Could you check a few things on this model? Use its own coordinates, in mm. A direction names the side the tool comes from. Coordinates: 2 decimals unless noted, no trailing zeros. Order: outer loops, then holes, each group sorted by start corner. A loop starts at its lowest first (then second) coordinate and runs counter-clockwise, first axis right, second up. Notation, with made-up numbers: (49.25, 34.25) -> (57.25, 34.25) arc R26 cw to (57.25, 57.25) -> close; hole circle Ø11 at (60, 55.5). An arc over 180 degrees is marked (long way). Put each result on its own line as item: value. Start each with the question number.
Q1. Please list where these lines run through material, in increasing order: line 1 along X through (y, z) = (31, -1.9); line 2 along X through (y, z) = (29, -0.2); line 3 along Y through (x, z) = (-52, -2.9).
Q2. We'd pull the mould along X, two halves only. Please class faces 1 (the face through (0, 15, -2)), 2 (the face through (-21.74, 14.93, -1.61)), 3 (the face through (-80, 33, 0)): +X half, -X half, draft (parallel to the pull), parting line (faces both ways), or undercut.
Q3. If we section it at C-C (z = -0.9): Count the separate pieces of the cut face and the enclosed holes in it, and give its area (3 significant figures).
Q4. For faces 4 (the face through (-26.988, 42, -2)), 5 (the face through (-58.444, 35.435, -1.61)), which set-ups out of +Z, -Z, +X, -X, +Y, -Y let a thin tool reach every point of the face, with its end or its side?
Q5. If we section it at A-A (x = -35.56): Please give me the cut outline in (y, z) (3 decimals), and give its area (3 significant figures).
Q6. Will these pins go through, and if not, where does the flat tip stop? pin 1 (1.5 mm diameter, centred on y = 23.5, z = -2.5, fed in from -X); pin 2 (1.6 mm diameter, centred on x = -9.5, z = -1.5, fed in from +Y).
Q7. If we section it at B-B (y = 50.8): Please give me the cut outline in (x, z) (3 decimals).
Q8. If we section it at D-D (x = -125.5): Please give me the cut outline in (y, z) (3 decimals).
from build123d import *

# Parameters (mm, degrees)
BOSS_EXTRUDE1_DEPTH             = 3.175
F_1_2_0_5_DIAMETER_HOLE1_D      = 12.7
F_9_64_0_14063_DIAMETER_HOLE1_D = 3.572002
F_6_CLEARANCE_HOLE1_D           = 4.3053
F_6_CLEARANCE_HOLE2_D           = 4.3053


with BuildPart() as part:
    # Sketch1 → Boss-Extrude1 (new body)
    with BuildSketch(Plane.XY):
        with BuildLine():
            Line((-26.9875, 34.925), (-26.9875, 48.5775))
            Line((-26.9875, 48.5775), (-38.29743402, 59.88743402))
            Line((-38.29743402, 59.88743402), (-157.398586801, 65.087510963))
            Line((-157.398586801, 65.087510963), (-153.9875, 1.0725e-05))
            Line((-153.9875, 1.0725e-05), (0, 0))
            Line((0, 0), (0, 30.1625))
            Line((0, 30.1625), (-22.225, 30.1625))
            ThreePointArc((-22.225, 30.1625), (-25.592596045, 31.557403955), (-26.9875, 34.925))
        make_face()
    extrude(amount=-BOSS_EXTRUDE1_DEPTH)

    # 1/2 (0.5) Diameter Hole1 (through all)
    with Locations(Plane.XY):
        with Locations((-112.7125, 33.528), (-52.3875, 33.528)):
            Hole(F_1_2_0_5_DIAMETER_HOLE1_D / 2)

    # 9/64 (0.14063) Diameter Hole1 (through all)
    with Locations(Plane.XY):
        with Locations((-112.7125, 43.053), (-52.3875, 43.053)):
            Hole(F_9_64_0_14063_DIAMETER_HOLE1_D / 2)

    # #6 Clearance Hole1 (through all)
    with Locations(Plane.XY):
        with Locations((-133.35, 30.1625), (-35.56, 43.688)):
            Hole(F_6_CLEARANCE_HOLE1_D / 2)

    # #6 Clearance Hole2 (through all)
    with Locations(Plane.XY):
        with Locations((-138.1125, 50.8), (-19.685, 14.2875)):
            Hole(F_6_CLEARANCE_HOLE2_D / 2)


solid = part.part
The answers:
1. line 1: -155.61 to -135.33, -131.37 to -118.54, -106.89 to -58.21, -46.56 to -24.92
1. line 2: -155.51 to -135.16, -131.54 to -117.16, -108.26 to -56.84, -47.94 to 0
1. line 3: 0 to 27.19, 39.87 to 41.31, 44.8 to 60.49
2. face 1: +X half
2. face 2: undercut
2. face 3: draft
3. separate pieces: 1
3. enclosed holes: 8
3. area: 8,430 mm^2
4. face 4: +Z, -Z, +X, +Y
4. face 5: +Z, -Z
5. outline: (0, -3.175) -> (41.535, -3.175) -> (41.535, 0) -> (0, 0) -> close; (45.841, -3.175) -> (57.15, -3.175) -> (57.15, 0) -> (45.841, 0) -> close
5. area: 168 mm^2
6. pin 1: x = -155.26
6. pin 2: y = 30.16
7. outline: (-156.65, -3.175) -> (-140.265, -3.175) -> (-140.265, 0) -> (-156.65, 0) -> close; (-135.96, -3.175) -> (-29.21, -3.175) -> (-29.21, 0) -> (-135.96, 0) -> close
8. outline: (0, -3.175) -> (63.695, -3.175) -> (63.695, 0) -> (0, 0) -> close
